from build123d import *

# Parameters (mm, degrees)
SKETCH1_R           = 11
BOSS_EXTRUDE1_DEPTH = 15
SKETCH3_R           = 10
CUT_EXTRUDE1_DEPTH  = 11
SKETCH4_R           = 4.15
SKETCH4_R_2         = 1.25
CUT_EXTRUDE2_DEPTH  = 11


with BuildPart() as part:
    # Sketch1 → Boss-Extrude1 (new body)
    with BuildSketch(Plane.XY):
        Circle(SKETCH1_R)
    extrude(amount=BOSS_EXTRUDE1_DEPTH)

    # Sketch3 → Cut-Extrude1 (cut)
    with BuildSketch(Plane.XY.offset(15)):
        Circle(SKETCH3_R)
    extrude(amount=-CUT_EXTRUDE1_DEPTH, mode=Mode.SUBTRACT)

    # Sketch4 → Cut-Extrude2 (cut)
    with BuildSketch(Plane(origin=(0, 0, 0), x_dir=(-1, 0, 0), z_dir=(0, 0, -1))):
        Circle(SKETCH4_R)
        with Locations((0, 8)):
            Circle(SKETCH4_R_2)
        with Locations((5.656854249, 5.656854249)):
            Circle(SKETCH4_R_2)
        with Locations((8, 0)):
            Circle(SKETCH4_R_2)
        with Locations((5.656854249, -5.656854249)):
            Circle(SKETCH4_R_2)
        with Locations((0, -8)):
            Circle(SKETCH4_R_2)
        with Locations((-5.656854249, -5.656854249)):
            Circle(SKETCH4_R_2)
        with Locations((-8, 0)):
            Circle(SKETCH4_R_2)
        with Locations((-5.656854249, 5.656854249)):
            Circle(SKETCH4_R_2)
    extrude(amount=-CUT_EXTRUDE2_DEPTH, mode=Mode.SUBTRACT)


solid = part.part
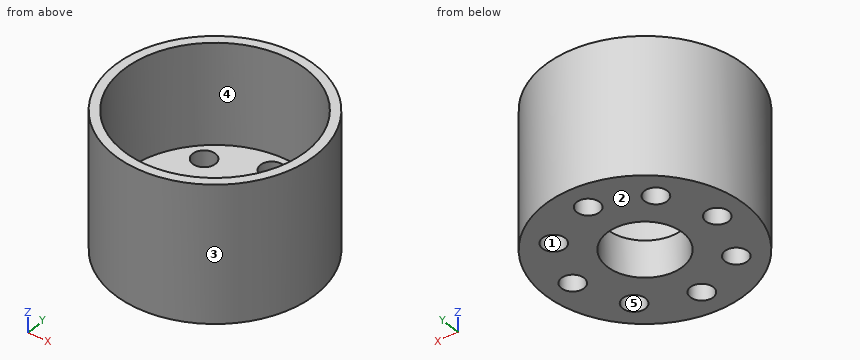
The listing builds one solid part. Answer for the finished solid, in the listing's coordinates (mm). Face numbers are marked on the shaded views. A direction names the side the tool comes from. Give positions to 0.01 mm unless a question says otherwise; leave off trailing zeros. Write each loop counter-clockwise with the first axis right and the second up, starting at its lowest first coordinate (ties: lowest second). Pieces come first, ordered by that corner, then holes.
Item 1: Section D-D, the plane y = 8 is taken. Write down the section's boundary in (x, z), plus the area to 3 significant figures.
Item 2: Section C-C, the plane x = 2.5 is taken. Write down the section's boundary in (y, z), plus the area to 3 significant figures.
Item 3: Determine the mould class of the marked faces 1, 2 and 3 for opening direction Y: released by +Y, released by -Y, zero draft, split by the parting line, or undercut.
Item 4: Flat-ended cylindrical pins translate along their axes: P1, Ø1, axis at y = 3, z = 13, coming from the +X side; P2, Ø1.5, axis at y = 8.5, z = 11, coming from the +X side; P3, Ø4, axis at x = 8, z = 13, coming from the -Y side. Find the tip coordinate at first contact, or state that the pin passes through.
Item 5: Find the intervals of material crossed by line 1 along Y through (x, z) = (0, 2.2); line 2 along Y through (x, z) = (0, 11); line 3 along Y through (x, z) = (0.5, 0.5), in increasing order.
Item 6: Section A-A, the plane x = 0 is taken. Write down the section's boundary in (y, z), plus the area to 3 significant figures.
Item 7: Which of the six approach directions +Z, -Z, +X, -X, +Y, -Y give full straight-line access (tool end or side, diameter ignored) to the marked faces 4 and 5?
Completed:
1. outline: (-7.55, 0) - (-1.25, 0) - (-1.25, 4) - (-6, 4) - (-6, 15) - (-7.55, 15) - close; (1.25, 0) - (7.55, 0) - (7.55, 15) - (6, 15) - (6, 4) - (1.25, 4) - close
1. area: 84.5 mm2
2. outline: (-10.71, 0) - (-3.31, 0) - (-3.31, 4) - (-9.68, 4) - (-9.68, 15) - (-10.71, 15) - close; (3.31, 0) - (10.71, 0) - (10.71, 15) - (9.68, 15) - (9.68, 4) - (3.31, 4) - close
2. area: 81.9 mm2
3. face 1: undercut
3. face 2: zero draft
3. face 3: split by the parting line
4. P1: stops at x = 10.71
4. P2: stops at x = 7.81
4. P3: stops at y = -9.22
5. line 1: y = -11 to -9.25, -6.75 to -4.15, 4.15 to 6.75, 9.25 to 11
5. line 2: y = -11 to -10, 10 to 11
5. line 3: y = -10.99 to -9.15, -6.85 to -4.12, 4.12 to 6.85, 9.15 to 10.99
6. outline: (-11, 0) - (-9.25, 0) - (-9.25, 4) - (-10, 4) - (-10, 15) - (-11, 15) - close; (-6.75, 0) - (-4.15, 0) - (-4.15, 4) - (-6.75, 4) - close; (4.15, 0) - (6.75, 0) - (6.75, 4) - (4.15, 4) - close; (9.25, 0) - (11, 0) - (11, 15) - (10, 15) - (10, 4) - (9.25, 4) - close
6. area: 56.8 mm2
7. face 4: +Z
7. face 5: +Z, -Z
